```python
from build123d import *

# Parameters (mm, degrees)
EXTRUDE_1_DEPTH = 6.5
EXTRUDE_START   = 6.5
EXTRUDE_2_DEPTH = 13
CHAMFER_9_SIZE  = 0.1
CHAMFER_1_SIZE  = 0.3


with BuildPart() as part:
    # ｽｹｯﾁ1 → ﾎﾞｽ - 押し出し1 (new body)
    with BuildSketch(Plane.XY):
        with BuildLine():
            ThreePointArc((0, 3.975), (-1.409787218, 3.71660127), (-2.636285265, 2.975))
            Line((-2.636285265, 2.975), (0, 2.975))
            Line((0, 2.975), (0, 3.975))
        make_face()
        with BuildLine():
            Line((0, 2.975), (-2.636285265, 2.975))
            ThreePointArc((-2.636285265, 2.975), (-3.71660127, -1.409787218), (0, -3.975))
            Line((0, -3.975), (0, 2.975))
        make_face()
        with BuildLine():
            Line((0, 3.975), (0, 2.975))
            Line((0, 2.975), (2.636285265, 2.975))
            ThreePointArc((2.636285265, 2.975), (1.409787218, 3.71660127), (0, 3.975))
        make_face()
        with BuildLine():
            Line((2.636285265, 2.975), (0, 2.975))
            Line((0, 2.975), (0, -3.975))
            ThreePointArc((0, -3.975), (2.810749455, -2.810749455), (3.975, 0))
            ThreePointArc((3.975, 0), (3.624904063, 1.631163859), (2.636285265, 2.975))
        make_face()
    extrude(amount=EXTRUDE_1_DEPTH)

    # ｽｹｯﾁ1<3> → ﾎﾞｽ - 押し出し2 (add)
    with BuildSketch(Plane.XY.offset(EXTRUDE_START)):
        with BuildLine():
            ThreePointArc((-2.636285265, 2.975), (0, -3.975), (2.636285265, 2.975))
            Line((2.636285265, 2.975), (-2.636285265, 2.975))
        make_face()
    extrude(amount=EXTRUDE_2_DEPTH)

    # 面取り9
    # the kernel refuses this chamfer: 0.1 mm, written as the material it takes off along each edge
    with BuildSketch(Plane(origin=(0, 0, 6.5), x_dir=(-0.7102313336903862, 0.7039683605421307, 0), z_dir=(-0.7039683605421307, -0.7102313336903862, 0))) as chamfer_9_piece_1_section:
        Polygon((3.975, CHAMFER_9_SIZE), (3.975 - CHAMFER_9_SIZE, 0), (3.975, 0), align=None)
    chamfer_9_piece_1 = revolve(axis=Axis((0, 0, 6.5), (0, 0, -1)), revolution_arc=90.507480781, mode=Mode.PRIVATE)
    chamfer_9_piece_1 = split(chamfer_9_piece_1, bisect_by=Plane(origin=(0, 2.975, 6.452222293), z_dir=(0, 1, 0)), keep=Keep.TOP, mode=Mode.PRIVATE)
    add(chamfer_9_piece_1, mode=Mode.SUBTRACT)
    with BuildSketch(Plane(origin=(2.893453564, 2.975, 19.5), x_dir=(0, 0.02749587661058671, -0.9996219169112966), z_dir=(-1, 0, 0))) as chamfer_9_piece_2:
        Polygon((CHAMFER_9_SIZE * 0.999621916911, CHAMFER_9_SIZE * 0.0274958766106), (-CHAMFER_9_SIZE * 0.0274958766106, CHAMFER_9_SIZE * 0.999621916911), (0, 0), align=None)
    extrude(amount=5.786907128, mode=Mode.SUBTRACT)

    # 面取り1
    chamfer_1_edges = [part.edges().sort_by_distance(p)[0] for p in [
        (0, -3.975, 19.5),
    ]]
    chamfer(chamfer_1_edges, length=CHAMFER_1_SIZE)


solid = part.part
```
CAD build for the part. Positions are in the model's coordinates, mm. A direction names the side the tool comes from. Round coordinates to 2 decimals unless told otherwise and drop trailing zeros. Order: outer loops, then holes, each group sorted by start corner. A loop starts at its lowest first (then second) coordinate and runs counter-clockwise, first axis right, second up. Notation, with made-up numbers: (29, -30.5) -> (53, -30.5) arc R27 cw to (53, -11.5) -> close; hole circle Ø10 at (-12, 81). An arc over 180 degrees is marked (long way). Write item = value, one per line.
(1) Flat gauge pins, fed straight in: P1, Ø1.6, axis at x = -0.5, z = 14, coming from the +Y side (3 decimals); P2, Ø4, axis at y = 2.5, z = 2, coming from the -X side; P3, Ø1, axis at y = 0.5, z = 8, coming from the -X side (3 decimals); P4, Ø2, axis at x = 2.5, z = 7, coming from the +Y side. Where does each tip first touch, or does it go through?
Answers follow:
P1 = 2.975
P2 = -3.94
P3 = -3.975
P4 = 3.59
(2) 3-axis set-ups, long thin cutter, end or side, ignore diameter. For faces 1 (the flat face through (0, 0, 0)), 2 (the flat face through (0, 3.3, 6.5)): which of +Z, -Z, +X, -X, +Y, -Y reach the whole face in a straight line?
Answers follow:
face_1 = -Z, +X, -X, +Y, -Y
face_2 = +Z, +X, -X, +Y
(3) Cut at A-A (z = 5). Write the cut outline in (x, y) (3 decimals).
Answers follow:
outline = circle Ø7.95 at (0, 0)
(4) Cut at B-B (z = 9). Write the cut outline in (x, y) (3 decimals), plus the area to 3 significant figures.
Answers follow:
outline = (-2.636, 2.975) arc R3.975 ccw (long way) to (2.636, 2.975) -> close
area = 46.0 mm²
(5) Drill centre lines: L1, parallel to Z at x = -0.75, y = 3.25; L2, parallel to Y at x = 1.75, z = 7 (3 decimals); L3, parallel to Y at x = -1.5, z = 11 (3 decimals). Where is each one in solid material? Low to high.
Answers follow:
L1 = 0 to 6.5
L2 = -3.569 to 2.975
L3 = -3.681 to 2.975
